Can you work these out from the model? Positions are in its coordinate system, mm. A direction names the side the tool comes from. Give positions to 0.01 mm unless a question says otherwise; leave off trailing zeros. Write each loop counter-clockwise with the first axis right and the second up, starting at its lowest first coordinate (ties: lowest second). Pieces come first, ordered by that corner, then holes.
```python
from build123d import *

# Parameters (mm, degrees)
SKETCH1_W           = 240
SKETCH1_H           = 116
BOSS_EXTRUDE1_DEPTH = 8
FILLET1_R           = 5
CUT_EXTRUDE1_REACH  = 135.522
SKETCH2_R           = 1.5
FILLET2_R           = 5
SKETCH3_R           = 3
SKETCH3_R_2         = 1.5
CUT_EXTRUDE2_DEPTH  = 2
SHELL1_DEPTH        = 3
SHELL1_2_DEPTH      = 1
CUT_EXTRUDE3_REACH  = 135.522
SKETCH4_R           = 3.5


# Read off the part's stored shape, not the designer's step: Shell1
with BuildPart() as part:
    # Sketch1 → Boss-Extrude1 (new body)
    with BuildSketch(Plane(origin=(0, 0, 0), x_dir=(1, 0, 0), z_dir=(0, 1, 0))):
        Rectangle(SKETCH1_W, SKETCH1_H)
    extrude(amount=BOSS_EXTRUDE1_DEPTH)

    # Fillet1
    fillet1_edges = [part.edges().sort_by_distance(p)[0] for p in [
        (120, 4, 58),
        (-120, 4, 58),
        (-120, 4, -58),
        (120, 4, -58),
    ]]
    fillet(fillet1_edges, radius=FILLET1_R)

    # Sketch2 → Cut-Extrude1 (cut, up to next)
    with BuildSketch(Plane(origin=(0, 8, 0), x_dir=(1, 0, 0), z_dir=(0, 1, 0)), mode=Mode.PRIVATE) as cut_extrude1_sk1:
        with Locations(Location((-115, -53, 0), (0, 0, 270))):
            Circle(SKETCH2_R)
    cut_extrude1_tool1 = extrude(cut_extrude1_sk1.sketch, amount=-CUT_EXTRUDE1_REACH, mode=Mode.PRIVATE) & part.part
    # Sketch2 → Cut-Extrude1 (cut, up to next)
    with BuildSketch(Plane(origin=(0, 8, 0), x_dir=(1, 0, 0), z_dir=(0, 1, 0)), mode=Mode.PRIVATE) as cut_extrude1_sk2:
        with Locations(Location((-115, 53, 0), (0, 0, 270))):
            Circle(SKETCH2_R)
    cut_extrude1_tool2 = extrude(cut_extrude1_sk2.sketch, amount=-CUT_EXTRUDE1_REACH, mode=Mode.PRIVATE) & part.part
    # Sketch2 → Cut-Extrude1 (cut, up to next)
    with BuildSketch(Plane(origin=(0, 8, 0), x_dir=(1, 0, 0), z_dir=(0, 1, 0)), mode=Mode.PRIVATE) as cut_extrude1_sk3:
        with Locations(Location((115, 53, 0), (0, 0, 270))):
            Circle(SKETCH2_R)
    cut_extrude1_tool3 = extrude(cut_extrude1_sk3.sketch, amount=-CUT_EXTRUDE1_REACH, mode=Mode.PRIVATE) & part.part
    # Sketch2 → Cut-Extrude1 (cut, up to next)
    with BuildSketch(Plane(origin=(0, 8, 0), x_dir=(1, 0, 0), z_dir=(0, 1, 0)), mode=Mode.PRIVATE) as cut_extrude1_sk4:
        with Locations(Location((115, -53, 0), (0, 0, 270))):
            Circle(SKETCH2_R)
    cut_extrude1_tool4 = extrude(cut_extrude1_sk4.sketch, amount=-CUT_EXTRUDE1_REACH, mode=Mode.PRIVATE) & part.part
    add(cut_extrude1_tool1.solids().sort_by_distance((-115, 8, 53))[0], mode=Mode.SUBTRACT)
    add(cut_extrude1_tool2.solids().sort_by_distance((-115, 8, -53))[0], mode=Mode.SUBTRACT)
    add(cut_extrude1_tool3.solids().sort_by_distance((115, 8, -53))[0], mode=Mode.SUBTRACT)
    add(cut_extrude1_tool4.solids().sort_by_distance((115, 8, 53))[0], mode=Mode.SUBTRACT)

    # Fillet2
    # the kernel refuses this fillet: 5 mm, written as the material it takes off along each edge
    with BuildSketch(Plane(origin=(-115, 8, -58), x_dir=(0, -1, 0), z_dir=(1, 0, 0))) as fillet2_piece_1:
        with BuildLine():
            CenterArc((FILLET2_R, -FILLET2_R), FILLET2_R, 90, 90)
            Line((0, -FILLET2_R), (0, 0))
            Line((0, 0), (FILLET2_R, 0))
        make_face()
    extrude(amount=230, mode=Mode.SUBTRACT)
    with BuildSketch(Plane(origin=(120, 8, -53), x_dir=(-1, 0, 0), z_dir=(0, 0, 1)), Plane(origin=(-120, 8, 53), x_dir=(1, 0, 0), z_dir=(0, 0, -1))) as fillet2_piece_2:
        with BuildLine():
            CenterArc((FILLET2_R, FILLET2_R), FILLET2_R, 180, 90)
            Line((0, FILLET2_R), (0, 0))
            Line((0, 0), (FILLET2_R, 0))
        make_face()
    extrude(amount=106, mode=Mode.SUBTRACT)
    with BuildSketch(Plane(origin=(115, 8, 58), x_dir=(0, 0, -1), z_dir=(-1, 0, 0))) as fillet2_piece_3:
        with BuildLine():
            CenterArc((FILLET2_R, FILLET2_R), FILLET2_R, 180, 90)
            Line((0, FILLET2_R), (0, 0))
            Line((0, 0), (FILLET2_R, 0))
        make_face()
    extrude(amount=230, mode=Mode.SUBTRACT)
    with BuildSketch(Plane(origin=(-115, 8, 53), x_dir=(0, 0, 1), z_dir=(1, 0, 0))) as fillet2_piece_4:
        with BuildLine():
            CenterArc((5 - FILLET2_R, FILLET2_R), FILLET2_R, 270, 90)
            Line((5, FILLET2_R), (5, 0))
            Line((5, 0), (5 - FILLET2_R, 0))
        make_face()
    revolve(axis=Axis((-115, 8, 53), (0, -1, 0)), revolution_arc=90, mode=Mode.SUBTRACT)
    with BuildSketch(Plane(origin=(-115, 8, -53), x_dir=(0, 0, -1), z_dir=(1, 0, 0))) as fillet2_piece_5:
        with BuildLine():
            CenterArc((5 - FILLET2_R, -FILLET2_R), FILLET2_R, 0, 90)
            Line((5 - FILLET2_R, 0), (5, 0))
            Line((5, 0), (5, -FILLET2_R))
        make_face()
    revolve(axis=Axis((-115, 8, -53), (0, 1, 0)), revolution_arc=90, mode=Mode.SUBTRACT)
    with BuildSketch(Plane(origin=(115, 8, 53), x_dir=(1, 0, 0), z_dir=(0, 0, -1))) as fillet2_piece_6:
        with BuildLine():
            CenterArc((5 - FILLET2_R, FILLET2_R), FILLET2_R, 270, 90)
            Line((5, FILLET2_R), (5, 0))
            Line((5, 0), (5 - FILLET2_R, 0))
        make_face()
    revolve(axis=Axis((115, 8, 53), (0, -1, 0)), revolution_arc=90, mode=Mode.SUBTRACT)
    with BuildSketch(Plane(origin=(115, 8, -53), x_dir=(0, 0, -1), z_dir=(-1, 0, 0))) as fillet2_piece_7:
        with BuildLine():
            CenterArc((5 - FILLET2_R, FILLET2_R), FILLET2_R, 270, 90)
            Line((5 - FILLET2_R, 0), (5, 0))
            Line((5, 0), (5, FILLET2_R))
        make_face()
    revolve(axis=Axis((115, 8, -53), (0, -1, 0)), revolution_arc=90, mode=Mode.SUBTRACT)

    # Sketch3 → Cut-Extrude2 (cut)
    # profile 1 of 4: a face of its own
    with BuildSketch(Plane(origin=(0, 8, 0), x_dir=(1, 0, 0), z_dir=(0, 1, 0))):
        with Locations(Location((-115, 53, 0), (0, 0, 270))):
            Circle(SKETCH3_R)
        with Locations(Location((-115, 53, 0), (0, 0, 270))):
            Circle(SKETCH3_R_2, mode=Mode.SUBTRACT)
    # profile 2 of 4: a face of its own
    with BuildSketch(Plane(origin=(0, 8, 0), x_dir=(1, 0, 0), z_dir=(0, 1, 0))):
        with Locations(Location((-115, -53, 0), (0, 0, 90))):
            Circle(SKETCH3_R)
        with Locations(Location((-115, -53, 0), (0, 0, 270))):
            Circle(SKETCH3_R_2, mode=Mode.SUBTRACT)
    # profile 3 of 4: a face of its own
    with BuildSketch(Plane(origin=(0, 8, 0), x_dir=(1, 0, 0), z_dir=(0, 1, 0))):
        with Locations(Location((115, -53, 0), (0, 0, 270))):
            Circle(SKETCH3_R)
        with Locations(Location((115, -53, 0), (0, 0, 270))):
            Circle(SKETCH3_R_2, mode=Mode.SUBTRACT)
    # profile 4 of 4: a face of its own
    with BuildSketch(Plane(origin=(0, 8, 0), x_dir=(1, 0, 0), z_dir=(0, 1, 0))):
        with Locations(Location((115, 53, 0), (0, 0, 90))):
            Circle(SKETCH3_R)
        with Locations(Location((115, 53, 0), (0, 0, 270))):
            Circle(SKETCH3_R_2, mode=Mode.SUBTRACT)
    extrude(amount=-CUT_EXTRUDE2_DEPTH, mode=Mode.SUBTRACT)

    # Shell1 outline → Shell1 (cut)
    with BuildSketch(Plane(origin=(0, 0, 0), x_dir=(1, 0, 0), z_dir=(0, 1, 0))):
        with BuildLine():
            ThreePointArc((-107, 53), (-109.343145751, 47.343145751), (-115, 45))
            Line((-115, 45), (-115, -45))
            ThreePointArc((-115, -45), (-109.343145751, -47.343145751), (-107, -53))
            Line((-107, -53), (107, -53))
            ThreePointArc((107, -53), (109.343145751, -47.343145751), (115, -45))
            Line((115, -45), (115, 45))
            ThreePointArc((115, 45), (109.343145751, 47.343145751), (107, 53))
            Line((107, 53), (-107, 53))
        make_face()
    extrude(amount=SHELL1_DEPTH, mode=Mode.SUBTRACT)

    # Shell1 2 outline → Shell1 2 (cut)
    with BuildSketch(Plane(origin=(0, 0, 0), x_dir=(1, 0, 0), z_dir=(0, 1, 0))):
        with BuildLine():
            Line((-115, 46.5), (-115, 45))
            ThreePointArc((-115, 45), (-109.343145751, 47.343145751), (-107, 53))
            Line((-107, 53), (-108.5, 53))
            ThreePointArc((-108.5, 53), (-110.403805922, 48.403805922), (-115, 46.5))
        make_face()
        with BuildLine():
            ThreePointArc((-107, -53), (-109.343145751, -47.343145751), (-115, -45))
            Line((-115, -45), (-115, -46.5))
            ThreePointArc((-115, -46.5), (-110.403805922, -48.403805922), (-108.5, -53))
            Line((-108.5, -53), (-107, -53))
        make_face()
        with BuildLine():
            Line((108.5, 53), (107, 53))
            ThreePointArc((107, 53), (109.343145751, 47.343145751), (115, 45))
            Line((115, 45), (115, 46.5))
            ThreePointArc((115, 46.5), (110.403805922, 48.403805922), (108.5, 53))
        make_face()
        with BuildLine():
            ThreePointArc((115, -45), (109.343145751, -47.343145751), (107, -53))
            Line((107, -53), (108.5, -53))
            ThreePointArc((108.5, -53), (110.403805922, -48.403805922), (115, -46.5))
            Line((115, -46.5), (115, -45))
        make_face()
    extrude(amount=SHELL1_2_DEPTH, mode=Mode.SUBTRACT)

    # Sketch4 → Cut-Extrude3 (cut, up to next)
    with BuildSketch(Plane(origin=(0, 8, 0), x_dir=(1, 0, 0), z_dir=(0, 1, 0)), mode=Mode.PRIVATE) as cut_extrude3_sk1:
        with Locations(Location((24, 0, 0), (0, 0, 270))):
            Circle(SKETCH4_R)
    cut_extrude3_tool1 = extrude(cut_extrude3_sk1.sketch, amount=-CUT_EXTRUDE3_REACH, mode=Mode.PRIVATE) & part.part
    # Sketch4 → Cut-Extrude3 (cut, up to next)
    with BuildSketch(Plane(origin=(0, 8, 0), x_dir=(1, 0, 0), z_dir=(0, 1, 0)), mode=Mode.PRIVATE) as cut_extrude3_sk2:
        with Locations(Location((50, 26, 0), (0, 0, 270))):
            Circle(SKETCH4_R)
    cut_extrude3_tool2 = extrude(cut_extrude3_sk2.sketch, amount=-CUT_EXTRUDE3_REACH, mode=Mode.PRIVATE) & part.part
    # Sketch4 → Cut-Extrude3 (cut, up to next)
    with BuildSketch(Plane(origin=(0, 8, 0), x_dir=(1, 0, 0), z_dir=(0, 1, 0)), mode=Mode.PRIVATE) as cut_extrude3_sk3:
        with Locations(Location((76, 0, 0), (0, 0, 270))):
            Circle(SKETCH4_R)
    cut_extrude3_tool3 = extrude(cut_extrude3_sk3.sketch, amount=-CUT_EXTRUDE3_REACH, mode=Mode.PRIVATE) & part.part
    # Sketch4 → Cut-Extrude3 (cut, up to next)
    with BuildSketch(Plane(origin=(0, 8, 0), x_dir=(1, 0, 0), z_dir=(0, 1, 0)), mode=Mode.PRIVATE) as cut_extrude3_sk4:
        with Locations(Location((50, -26, 0), (0, 0, 270))):
            Circle(SKETCH4_R)
    cut_extrude3_tool4 = extrude(cut_extrude3_sk4.sketch, amount=-CUT_EXTRUDE3_REACH, mode=Mode.PRIVATE) & part.part
    add(cut_extrude3_tool1.solids().sort_by_distance((24, 8, 0))[0], mode=Mode.SUBTRACT)
    add(cut_extrude3_tool2.solids().sort_by_distance((50, 8, -26))[0], mode=Mode.SUBTRACT)
    add(cut_extrude3_tool3.solids().sort_by_distance((76, 8, 0))[0], mode=Mode.SUBTRACT)
    add(cut_extrude3_tool4.solids().sort_by_distance((50, 8, 26))[0], mode=Mode.SUBTRACT)


solid = part.part
```
1) Suppose I cut it at A-A on x = 50. Write out the boundary of the cut face in (y, z), plus the area to 3 significant figures.
Values follow:
outline: (0, -58) - (3, -58) arc R5 ccw to (8, -53) - (8, -29.5) - (3, -29.5) - (3, -53) - (0, -53) - close; (0, 53) - (3, 53) - (3, 29.5) - (8, 29.5) - (8, 53) arc R5 ccw to (3, 58) - (0, 58) - close; (3, -22.5) - (8, -22.5) - (8, 22.5) - (3, 22.5) - close
area: 529 mm2
2) For faces 1 (the face through (-119, 2, 56)), 2 (the face through (-109.406, 1.986, 47.281)), 3 (the face through (113.2, 6.8, 50.6)), which set-ups out of +Z, -Z, +X, -X, +Y, -Y let a thin tool reach every point of the face, with its end or its side?
Values follow:
face 1: +Z, -X, +Y, -Y
face 2: -Y
face 3: +Y
3) Suppose I cut it at B-B on z = 0. Write out the boundary of the cut face in (x, y), plus the area to 3 significant figures.
Values follow:
outline: (-120, 0) - (-115, 0) - (-115, 3) - (20.5, 3) - (20.5, 8) - (-115, 8) arc R5 ccw to (-120, 3) - close; (27.5, 3) - (72.5, 3) - (72.5, 8) - (27.5, 8) - close; (79.5, 3) - (115, 3) - (115, 0) - (120, 0) - (120, 3) arc R5 ccw to (115, 8) - (79.5, 8) - close
area: 1,150 mm2
4) Please list where these lines run through material, in increasing order: L1, parallel to X at y = 3.05, z = -53; L2, parallel to X at y = 2.75, z = 12.5; L3, parallel to Z at x = -53.5, y = 2.75.
Values follow:
L1: x = -120 to -116.5, -113.5 to 113.5, 116.5 to 120
L2: x = -120 to -115, 115 to 120
L3: z = -58 to -53, 53 to 58
5) For pin 1 Ø1.5 at (x, z) = (-93.5, 40) entering from -Y; pin 2 Ø5 at (x, z) = (-115, -53) entering from +Y, each with a flat end and sliding along its axis, tell me the tip position at first contact or that it passes through.
Values follow:
pin 1: stops at y = 3
pin 2: stops at y = 6
6) Suppose I cut it at D-D on x = 76. Write out the boundary of the cut face in (y, z), plus the area to 3 significant figures.
Values follow:
outline: (0, -58) - (3, -58) arc R5 ccw to (8, -53) - (8, -3.5) - (3, -3.5) - (3, -53) - (0, -53) - close; (0, 53) - (3, 53) - (3, 3.5) - (8, 3.5) - (8, 53) arc R5 ccw to (3, 58) - (0, 58) - close
area: 564 mm2
7) Suppose I cut it at C-C on z = 26. Write out the boundary of the cut face in (x, y), plus the area to 3 significant figures.
Values follow:
outline: (-120, 0) - (-115, 0) - (-115, 3) - (46.5, 3) - (46.5, 8) - (-115, 8) arc R5 ccw to (-120, 3) - close; (53.5, 3) - (115, 3) - (115, 0) - (120, 0) - (120, 3) arc R5 ccw to (115, 8) - (53.5, 8) - close
area: 1,180 mm2
